```python
from build123d import *

# Parameters (mm, degrees)
SIDE_BOSS_SKETCH_W      = 18
SIDE_BOSS_SKETCH_H      = 16
SIDE_BOSS_DEPTH         = 9
SIDE_BOSS_2_SKETCH_W    = 18
SIDE_BOSS_2_SKETCH_H    = 16
SIDE_BOSS_2_DEPTH       = 9
BOTTOM_PORT_SKETCH_W    = 11.5
BOTTOM_PORT_SKETCH_H    = 4.953
SIDE_PORT_SKETCH_W      = 4.953
SIDE_PORT_SKETCH_H      = 11.5
SIDE_PASSAGE_SKETCH_W   = 2
SIDE_PASSAGE_SKETCH_H   = 5.5
SIDE_PORT_2_SKETCH_W    = 4.953
SIDE_PORT_2_SKETCH_H    = 11.5
SIDE_PASSAGE_2_SKETCH_W = 2
SIDE_PASSAGE_2_SKETCH_H = 5.5


with BuildPart() as part:
    # Reg_Outlet_Adapter Sketch → Reg_Outlet_Adapter (revolve)
    with BuildSketch(Plane.XY, mode=Mode.PRIVATE) as reg_outlet_adapter_sk:
        Polygon((14, 0), (14, 10), (0, 10), (0, 15), (-24, 15), (-24, 0), align=None)
    revolve(reg_outlet_adapter_sk.sketch.rotate(Axis((-1000, 0, 0), (1, 0, 0)), 90), axis=Axis((-1000, 0, 0), (1, 0, 0)))

    # Side Boss Sketch → Side Boss (add, symmetric)
    with BuildSketch(Plane.XY):
        with Locations((-12, 8)):
            Rectangle(SIDE_BOSS_SKETCH_W, SIDE_BOSS_SKETCH_H)
    extrude(amount=SIDE_BOSS_DEPTH, both=True)

    # Side Boss 2 Sketch → Side Boss 2 (add, symmetric)
    with BuildSketch(Plane.XY):
        with Locations((-12, -8)):
            Rectangle(SIDE_BOSS_2_SKETCH_W, SIDE_BOSS_2_SKETCH_H)
    extrude(amount=SIDE_BOSS_2_DEPTH, both=True)

    # Bottom Port Sketch → Bottom Port (revolve, cut)
    with BuildSketch(Plane.XY, mode=Mode.PRIVATE) as bottom_port_sk:
        with Locations((-19.25, 2.4765)):
            Rectangle(BOTTOM_PORT_SKETCH_W, BOTTOM_PORT_SKETCH_H)
    revolve(bottom_port_sk.sketch.rotate(Axis((-1000, 0, 0), (1, 0, 0)), 90), axis=Axis((-1000, 0, 0), (1, 0, 0)), mode=Mode.SUBTRACT)

    # Side Port Sketch → Side Port (revolve, cut)
    with BuildSketch(Plane.XY, mode=Mode.PRIVATE) as side_port_sk:
        with Locations((-9.5235, 11.25)):
            Rectangle(SIDE_PORT_SKETCH_W, SIDE_PORT_SKETCH_H)
    revolve(side_port_sk.sketch.rotate(Axis((-12, -60, 0), (0, 1, 0)), 90), axis=Axis((-12, -60, 0), (0, 1, 0)), mode=Mode.SUBTRACT)

    # Side Passage Sketch → Side Passage (revolve, cut)
    with BuildSketch(Plane.XY, mode=Mode.PRIVATE) as side_passage_sk:
        with Locations((-11, 2.75)):
            Rectangle(SIDE_PASSAGE_SKETCH_W, SIDE_PASSAGE_SKETCH_H)
    revolve(side_passage_sk.sketch.rotate(Axis((-12, -60, 0), (0, 1, 0)), 90), axis=Axis((-12, -60, 0), (0, 1, 0)), mode=Mode.SUBTRACT)

    # Side Port 2 Sketch → Side Port 2 (revolve, cut)
    with BuildSketch(Plane.XY, mode=Mode.PRIVATE) as side_port_2_sk:
        with Locations((-9.5235, -11.25)):
            Rectangle(SIDE_PORT_2_SKETCH_W, SIDE_PORT_2_SKETCH_H)
    revolve(side_port_2_sk.sketch.rotate(Axis((-12, -60, 0), (0, 1, 0)), 90), axis=Axis((-12, -60, 0), (0, 1, 0)), mode=Mode.SUBTRACT)

    # Side Passage 2 Sketch → Side Passage 2 (revolve, cut)
    with BuildSketch(Plane.XY, mode=Mode.PRIVATE) as side_passage_2_sk:
        with Locations((-11, -2.75)):
            Rectangle(SIDE_PASSAGE_2_SKETCH_W, SIDE_PASSAGE_2_SKETCH_H)
    revolve(side_passage_2_sk.sketch.rotate(Axis((-12, -60, 0), (0, 1, 0)), 90), axis=Axis((-12, -60, 0), (0, 1, 0)), mode=Mode.SUBTRACT)


solid = part.part
```
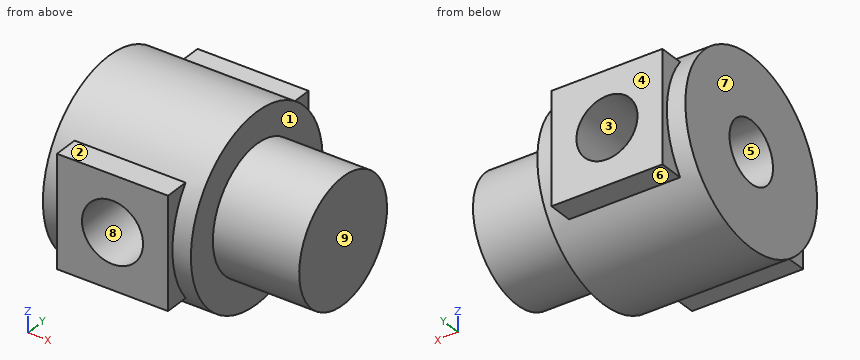
The listing builds one solid part. Answer for the finished solid, in the listing's coordinates (mm). Face numbers are marked on the shaded views. A direction names the side the tool comes from. Coordinates: 2 decimals unless noted, no trailing zeros. Loops run counter-clockwise (first coordinate to the right, second up) from the corner with the lowest first, then second, coordinate; pieces in that order, holes last. Notation, with made-up numbers: (19, -30) -> (27, -30) arc R24 ccw to (27, -16) -> close; hole circle Ø11 at (-19, 42). An arc over 180 degrees is marked (long way). Return JSON: item names as keys, results as strings. Group by question number.
(1) Determine the mould class of the marked faces 6, 7, 8 and 9 for opening direction X: released by +X, released by -X, zero draft, split by the parting line, or undercut.
(2) A cutting plane is placed at A-A on x = -12. Write down the section's boundary in (y, z).
(3) A cutting plane is placed at D-D on y = 12.5. Write down the section's boundary in (x, z), and give its area (3 significant figures).
(4) Find the intervals of material crossed by probe 1 along X at (y, z) = (10.5, 0); probe 2 along Y at (x, z) = (-20, 0); probe 3 along X at (y, z) = (-8, 0), in increasing order. Write a range as from..to.
(5) Given pin 1 Ø2 at (x, z) = (9.5, -1.5) entering from +Y; pin 2 Ø3 at (y, z) = (-14.5, -3.5) entering from +X; pin 3 Ø10 at (x, y) = (3.5, -6.5) entering from +Z, each flat-ended and moving along its own axis, determine where each tip first touches the part or whether it passes through.
(6) A cutting plane is placed at B-B on z = 0. Count the separate pieces of the cut face and the enclosed holes in it, and give its area (3 significant figures).
(7) Which of the six approach directions +Z, -Z, +X, -X, +Y, -Y give full straight-line access (tool end or side, diameter ignored) to the marked faces 1, 2, 3, 4 and 5?
(8) A cutting plane is placed at C-C on x = -6.5. Write down the section's boundary in (y, z), and give its area (3 significant figures).
The answers:
{
 "1": {"face 6": "zero draft", "face 7": "released by -X", "face 8": "undercut", "face 9": "released by +X"},
 "2": {"outline": "(-16, -9) -> (-12, -9) arc R15 ccw to (12, -9) -> (16, -9) -> (16, -4.95) -> (5.5, -4.95) -> (5.5, -2) -> (-5.5, -2) -> (-5.5, -4.95) -> (-16, -4.95) -> close; (-16, 4.95) -> (-5.5, 4.95) -> (-5.5, 2) -> (5.5, 2) -> (5.5, 4.95) -> (16, 4.95) -> (16, 9) -> (12, 9) arc R15 ccw to (-12, 9) -> (-16, 9) -> close"},
 "3": {"outline": "(-24, -8.29) -> (-21, -8.29) -> (-21, -9) -> (-3, -9) -> (-3, -8.29) -> (0, -8.29) -> (0, 8.29) -> (-3, 8.29) -> (-3, 9) -> (-21, 9) -> (-21, 8.29) -> (-24, 8.29) -> close; hole circle Ø9.91 at (-12, 0)", "area": "346 mm^2"},
 "4": {"probe 1": "x = -24..-16.95, -7.05..0", "probe 2": "y = -16..-4.95, 4.95..16", "probe 3": "x = -24..-16.95, -7.05..14"},
 "5": {"pin 1": "stops at y = 9.99", "pin 2": "stops at x = 0", "pin 3": "stops at z = 14.71"},
 "6": {"separate pieces": "3", "enclosed holes": "0", "area": "685 mm^2"},
 "7": {"face 1": "+X", "face 2": "+Z, +X, -X, -Y", "face 3": "+Y", "face 4": "+Z, -Z, +X, -X, +Y", "face 5": "-X"},
 "8": {"outline": "(-16, -9) -> (-12, -9) arc R15 ccw to (12, -9) -> (16, -9) -> (16, 9) -> (12, 9) arc R15 ccw to (-12, 9) -> (-16, 9) -> close", "area": "777 mm^2"}
}
